```python
from build123d import *

# Parameters (mm, degrees)
F1_DEPTH = 27
F2_DEPTH = 3


with BuildPart() as f1:
    # F0 (on Front) → F1 (new body)
    with BuildSketch(Plane.XZ):
        with BuildLine():
            ThreePointArc((1.456403, 9.893376), (0, -10), (-1.456403, 9.893376))
            Line((-1.456403, 9.893376), (-1.456403, 12.414866))
            ThreePointArc((-1.456403, 12.414866), (0, -12.5), (1.456403, 12.414866))
            Line((1.456403, 12.414866), (1.456403, 9.893376))
        make_face()
    extrude(amount=F1_DEPTH)

    # F0 (on Front) → F2 (join)
    with BuildSketch(Plane.XZ):
        with BuildLine():
            ThreePointArc((1.456403, 12.414866), (0, -12.5), (-1.456403, 12.414866))
            Line((-1.456403, 12.414866), (-1.456403, 14.929129))
            ThreePointArc((-1.456403, 14.929129), (0, -15), (1.456403, 14.929129))
            Line((1.456403, 14.929129), (1.456403, 12.414866))
        make_face()
    extrude(amount=F2_DEPTH)


solid = f1.part
```
CAD build for the part. Positions are in the model's coordinates, mm. A direction names the side the tool comes from. Coordinates: 2 decimals unless noted, no trailing zeros. Order: outer loops, then holes, each group sorted by start corner. A loop starts at its lowest first (then second) coordinate and runs counter-clockwise, first axis right, second up. Notation, with made-up numbers: (33, 28) - (79, 28) arc R24 cw to (79, 57) - close; hole circle Ø9 at (-8, -18). An arc over 180 degrees is marked (long way). Use a Markdown table: item, result. Add a question column.
(1) Saw through at C-C (y = -13.25). Give the cut face in (x, z), then the cut area to 3 significant figures.
(2) Flat gauge pins, fed straight in: pin 1 (8 mm diameter, centred on y = -24, z = -9, fed in from -X); pin 2 (5.5 mm diameter, centred on y = -18.5, z = 12.5, fed in from -X); pin 3 (2 mm diameter, centred on y = -14.5, z = 11.5, fed in from +X). Where does each tip first touch, or does it go through?
(3) Pull direction X, two halves, no side cores. Call faces 1 (the face through (-1.456, -13, 11)), 2 (the face through (1.456, -13, 11)), 3 (the face through (-0.98, -27, -10.13)), 4 (the face through (-0.53, -14.83, -12.49)): +X half, -X half, draft (parallel to the pull), parting line (faces both ways), or undercut.
(4) Saw through at D-D (z = -10.75). Give the cut face in (x, y), then the cut area to 3 significant figures.
(5) Which spindle directions (+Z, -Z, +X, -X, +Y, -Y) get a long thin tool onto all of the face, cutting with end or side? Do faces 5 (the face through (-3.4, -3, -12.2)), 6 (the face through (-0.639, -1.479, -14.986)). Say none if no direction does.
(6) Drill centre lines: line 1 along X through (y, z) = (-14.25, 0); line 2 along X through (y, z) = (-8.5, 2.5); line 3 along Z through (x, y) = (-5.5, -11.75). Where is each one in solid material? Low to high. Write a range as [from, to].
(7) Saw through at B-B (x = 3). Give the cut face in (y, z).
(8) Saw through at A-A (z = 0). Give the cut face in (x, y).
Solved:
| question | item | result |
|---|---|---|
| 1 | outline | (-1.46, 9.89) - (-1.46, 12.41) arc R12.5 ccw (long way) to (1.46, 12.41) - (1.46, 9.89) arc R10 cw (long way) to start |
| 1 | area | 169 mm² |
| 2 | pin 1 | stops at x = -11.46 |
| 2 | pin 2 | stops at x = -7.82 |
| 2 | pin 3 | stops at x = 6.78 |
| 3 | face 1 | undercut |
| 3 | face 2 | undercut |
| 3 | face 3 | draft |
| 3 | face 4 | parting line |
| 4 | outline | (-10.46, -3) - (-6.38, -3) - (-6.38, -27) - (6.38, -27) - (6.38, -3) - (10.46, -3) - (10.46, 0) - (-10.46, 0) - close |
| 4 | area | 369 mm² |
| 5 | face 5 | -Y |
| 5 | face 6 | +Y, -Y |
| 6 | line 1 | x = [-12.5, -10], [10, 12.5] |
| 6 | line 2 | x = [-12.25, -9.68], [9.68, 12.25] |
| 6 | line 3 | z = [-11.22, -8.35], [8.35, 11.22] |
| 7 | outline | (-27, -12.13) - (-3, -12.13) - (-3, -14.7) - (0, -14.7) - (0, -9.54) - (-27, -9.54) - close; (-27, 9.54) - (0, 9.54) - (0, 14.7) - (-3, 14.7) - (-3, 12.13) - (-27, 12.13) - close |
| 8 | outline | (-15, -3) - (-12.5, -3) - (-12.5, -27) - (-10, -27) - (-10, 0) - (-15, 0) - close; (10, -27) - (12.5, -27) - (12.5, -3) - (15, -3) - (15, 0) - (10, 0) - close |
